from build123d import *

# Parameters (mm, degrees)
SKETCH1_W                       = 95
SKETCH1_H                       = 95
SKETCH1_W_2                     = 81
SKETCH1_H_2                     = 81
SKETCH1_R                       = 40.1
BOSS_EXTRUDE1_DEPTH             = 5
F_4_0MM_DOWEL_HOLE1_D           = 4
BOSS_EXTRUDE2_DEPTH             = 3
FILLET1_R                       = 5
SKETCH6_W                       = 3
SKETCH6_H                       = 5
SKETCH6_W_2                     = 4.8
BOSS_EXTRUDE3_DEPTH             = 10
TAP_DRILL_FOR_M5X0_8_TAP1_D     = 4.2
TAP_DRILL_FOR_M5X0_8_TAP1_DEPTH = 12
TAP_DRILL_FOR_M5X0_8_TAP1_TIP   = 1.2618073
CHAMFER1_SIZE                   = 10


with BuildPart() as part:
    # Sketch1 → Boss-Extrude1 (new body)
    # profile 1 of 2: a face of its own
    with BuildSketch(Plane(origin=(0, 0, 0), x_dir=(1, 0, 0), z_dir=(0, 1, 0))):
        Rectangle(SKETCH1_W, SKETCH1_H)
        Rectangle(SKETCH1_W_2, SKETCH1_H_2, mode=Mode.SUBTRACT)
    # profile 2 of 2: a face of its own
    with BuildSketch(Plane(origin=(0, 0, 0), x_dir=(1, 0, 0), z_dir=(0, 1, 0))):
        Rectangle(SKETCH1_W_2, SKETCH1_H_2)
        with Locations(Location((0, 0, 0), (0, 0, 270))):
            Circle(SKETCH1_R, mode=Mode.SUBTRACT)
    extrude(amount=BOSS_EXTRUDE1_DEPTH)

    # Ø4.0mm Dowel Hole1 (through all)
    with Locations(Plane(origin=(0, 0, 0), x_dir=(-1, 0, 0), z_dir=(0, -1, 0))):
        with Locations((40.5, -40.5), (-40.5, -40.5), (-40.5, 40.5), (40.5, 40.5)):
            Hole(F_4_0MM_DOWEL_HOLE1_D / 2)

    # Sketch5 → Boss-Extrude2 (add)
    with BuildSketch(Plane.ZY.offset(47.5)):
        Polygon((0, 0), (-2.886751346, 5), (2.886751346, 5), align=None)
    extrude(amount=BOSS_EXTRUDE2_DEPTH)

    # Fillet1
    fillet1_edges = [part.edges().sort_by_distance(p)[0] for p in [
        (-47.5, 2.5, 47.5),
        (-47.5, 2.5, -47.5),
        (47.5, 2.5, -47.5),
        (47.5, 2.5, 47.5),
    ]]
    fillet(fillet1_edges, radius=FILLET1_R)

    # Sketch6 → Boss-Extrude3 (add)
    with BuildSketch(Plane(origin=(47.5, 0, 0), x_dir=(0, 0, -1), z_dir=(1, 0, 0))):
        with Locations((-1.5, 2.5)):
            Rectangle(SKETCH6_W, SKETCH6_H)
        with Locations((2.4, 2.5)):
            Rectangle(SKETCH6_W_2, SKETCH6_H)
        with Locations((6.3, 2.5)):
            Rectangle(SKETCH6_W, SKETCH6_H)
    extrude(amount=BOSS_EXTRUDE3_DEPTH)

    # Tap Drill for M5x0.8 Tap1
    with Locations(Plane(origin=(0, 5, 0), x_dir=(1, 0, 0), z_dir=(0, 1, 0))):
        with Locations((50.782954503, 2)):
            Hole(TAP_DRILL_FOR_M5X0_8_TAP1_D / 2, depth=TAP_DRILL_FOR_M5X0_8_TAP1_DEPTH)
            with Locations((0, 0, -(TAP_DRILL_FOR_M5X0_8_TAP1_DEPTH + TAP_DRILL_FOR_M5X0_8_TAP1_TIP / 2))):  # 118° drill point
                Cone(0, TAP_DRILL_FOR_M5X0_8_TAP1_D / 2, TAP_DRILL_FOR_M5X0_8_TAP1_TIP, mode=Mode.SUBTRACT)

    # Chamfer1
    chamfer1_edges = [part.edges().sort_by_distance(p)[0] for p in [
        (47.5, 2.5, 3),
        (47.5, 2.5, -7.8),
    ]]
    chamfer(chamfer1_edges, length=CHAMFER1_SIZE - 0.0001)  # a hair under: the kernel refuses the full size


solid = part.part
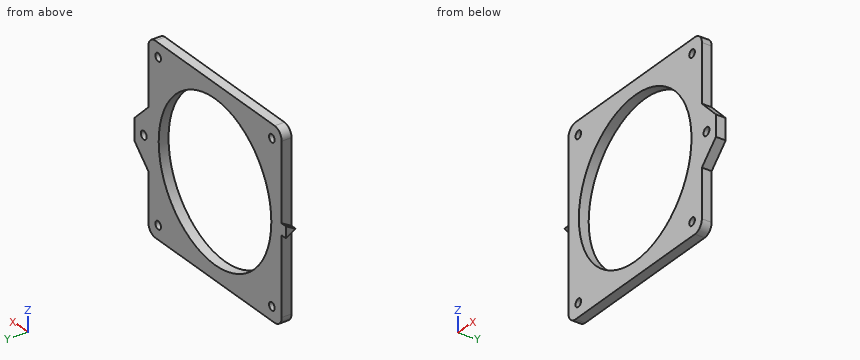
The model under review builds one solid part; all positions refer to its coordinate system, in mm. Round coordinates to 2 decimals unless told otherwise and drop trailing zeros. Write each loop counter-clockwise with the first axis right and the second up, starting at its lowest first coordinate (ties: lowest second). Pieces come first, ordered by that corner, then holes. Notation, with made-up numbers: (63.25, -2) - (90.25, -2) arc R20 ccw to (90.25, 15) - close; hole circle Ø9 at (13, -24.75). An arc over 180 degrees is marked (long way). One line per item, written item: value. Start each with the question number.
1. Consider section C-C on y = 4.05. State how many separate pieces and enclosed holes the cut face has, and give its area (3 significant figures).
2. Clearance check with a flat-ended pin moving along its axis: P1, Ø2.5, axis at y = 3.5, z = -27.5, coming from the +X side. State where the tip first meets the part, or that it passes through.
3. Consider section A-A on x = 0. Write out the cut boundary in (y, z), and give its area (3 significant figures).
4. To check wall thickness, follow L1, parallel to X at y = 1.75, z = -40.5; L2, parallel to X at y = 3.55, z = 1. State the ranges of each line that lie inside material, in increasing order. Write a range as from..to.
5. Consider section B-B on z = 27. Write out the cut boundary in (x, y).
Checks:
1. separate pieces: 1
1. enclosed holes: 6
1. area: 4,110 mm^2
2. P1: stops at x = 47.5
3. outline: (0, -47.5) - (5, -47.5) - (5, -40.1) - (0, -40.1) - close; (0, 40.1) - (5, 40.1) - (5, 47.5) - (0, 47.5) - close
3. area: 74.0 mm^2
4. L1: x = -47.5..-42.5, -38.5..38.5, 42.5..47.5
4. L2: x = -50.5..-40.09, 40.09..57.5
5. outline: (-47.5, 0) - (-29.65, 0) - (-29.65, 5) - (-47.5, 5) - close; (29.65, 0) - (47.5, 0) - (47.5, 5) - (29.65, 5) - close
